from build123d import *

# Parameters (mm, degrees)
SKIZZE1_W                       = 108
SKIZZE1_H                       = 78
AUFSATZ_LINEAR_AUSTRAGEN1_DEPTH = 5
SKIZZE2_W                       = 102
SKIZZE2_H                       = 72
SCHNITT_LINEAR_AUSTRAGEN1_DEPTH = 3
SKIZZE3_R                       = 3
SCHNITT_LINEAR_AUSTRAGEN2_DEPTH = 3
SKIZZE4_R                       = 10
SKIZZE4_R_2                     = 3
AUFSATZ_LINEAR_AUSTRAGEN2_DEPTH = 25


with BuildPart() as part:
    # Skizze1 → Aufsatz-Linear austragen1 (new body)
    with BuildSketch(Plane.XY):
        with Locations((-34.920453515, 9.024489796)):
            Rectangle(SKIZZE1_W, SKIZZE1_H)
    extrude(amount=AUFSATZ_LINEAR_AUSTRAGEN1_DEPTH)

    # Skizze2 → Schnitt-Linear austragen1 (cut)
    with BuildSketch(Plane.XY.offset(5)):
        with Locations((-34.920453515, 9.024489796)):
            Rectangle(SKIZZE2_W, SKIZZE2_H)
    extrude(amount=-SCHNITT_LINEAR_AUSTRAGEN1_DEPTH, mode=Mode.SUBTRACT)

    # Skizze3 → Schnitt-Linear austragen2 (cut)
    with BuildSketch(Plane.XY.offset(2)):
        with Locations((-39.920453515, 9.024489796)):
            Circle(SKIZZE3_R)
        with Locations((-29.920453515, 9.024489796)):
            Circle(SKIZZE3_R)
    extrude(amount=-SCHNITT_LINEAR_AUSTRAGEN2_DEPTH, mode=Mode.SUBTRACT)

    # Skizze4 → Aufsatz-Linear austragen2 (add, along a direction that is not the sketch's normal)
    with BuildSketch(Plane(origin=(0, 0, 0), x_dir=(-1, 0, 0), z_dir=(0, 0, -1))):
        with Locations((34.920453515, 28.024489796)):
            Circle(SKIZZE4_R)
        with Locations((34.920453515, 28.024489796)):
            Circle(SKIZZE4_R_2, mode=Mode.SUBTRACT)
    extrude(amount=AUFSATZ_LINEAR_AUSTRAGEN2_DEPTH, dir=(0, -0.7071067811865538, -0.7071067811865414))


solid = part.part
The listing builds one solid part. Answer for the finished solid, in the listing's coordinates (mm). A direction names the side the tool comes from. Coordinates: 2 decimals unless noted, no trailing zeros. Order: outer loops, then holes, each group sorted by start corner. A loop starts at its lowest first (then second) coordinate and runs counter-clockwise, first axis right, second up.
Q1. Which of the six approach directions +Z, -Z, +X, -X, +Y, -Y give full straight-line access (tool end or side, diameter ignored) to faces 4 (the face through (19.08, 8, 2)), 5 (the face through (-35, 28, 0)), 6 (the face through (-37.06, 9.93, 1.01))?
Q2. Consider line 1 (Z direction, x = -19.5, y = 38.5); line 2 (X direction, y = 26.5, z = -2.5); line 3 (X direction, y = 41, z = 3.25). Determine where each line is inside the solid, lowest interval first.
Q3. For a pull along Y with two mould halves and no side action, classify faces 1 (the face through (-36, 48.024, 2)), 2 (the face through (-88.92, 8, 2)), 3 (the face through (-85.92, 9, 4)) as pulls with the +Y half, pulls with the -Y half, needs draft (parallel to the pull), parting line crosses it, or undercut.
Q4. Given P1, Ø6.5, axis at x = -35.5, y = 28, coming from the -Z side; P2, Ø4, axis at y = 20.5, z = -11.5, coming from the -X side; P3, Ø2, axis at x = -4.5, y = 27.5, coming from the +Z side; P4, Ø1, axis at y = 12.5, z = -3.5, coming from the -X side, each flat-ended and moving along its own axis, determine where each tip first touches the part or whether it passes through.
Q5. A cutting plane is placed at B-B, the plane x = -7.5. Write down the section's boundary in (y, z).
Q6. A cutting plane is placed at A-A, the plane y = -24. Write down the section's boundary in (x, z).
Answers follow:
1. face 4: +Z, -Z, +X, +Y, -Y
1. face 5: none
1. face 6: +Z
2. line 1: z = 0 to 2
2. line 2: x = -44.87 to -37.76, -32.08 to -24.97
2. line 3: x = -88.92 to -85.92, 16.08 to 19.08
3. face 1: pulls with the +Y half
3. face 2: needs draft
3. face 3: undercut
4. P1: stops at z = -13.26
4. P2: stops at x = -44.85
4. P3: stops at z = 2
4. P4: passes through
5. outline: (-29.98, 0) - (48.02, 0) - (48.02, 5) - (45.02, 5) - (45.02, 2) - (-26.98, 2) - (-26.98, 5) - (-29.98, 5) - close
6. outline: (-88.92, 0) - (19.08, 0) - (19.08, 5) - (16.08, 5) - (16.08, 2) - (-85.92, 2) - (-85.92, 5) - (-88.92, 5) - close
